Solid Edge part; units mm, degrees
sketch "Sketch1" plane through (0, 0, 0) normal (0, 0, 1) x (1, 0, 0)
  line L0 (-45.39, -6.825) -> (45.39, -6.825)
  line L1 (45.39, -6.825) -> (45.39, 6.825)
  line L2 (45.39, 6.825) -> (-45.39, 6.825)
  line L3 (-45.39, 6.825) -> (-45.39, -6.825)
  dimension "D1" = 45.39
  dimension "D2" = 45.39
extrude "Protrusion1" add sketch "Sketch1" along normal blind 1
sketch "Sketch2" plane through (0, 0, 1) normal (0, 0, 1) x (1, 0, 0)
  line L0 (-35.761, 0.4214) -> (-34.261, 0.4214)
  line L1 (-34.261, 0.4214) -> (-34.261, 6.4214)
  line L2 (-34.261, 6.4214) -> (-35.761, 6.4214)
  line L3 (-35.761, 6.4214) -> (-35.761, 0.4214)
  line L4 (-28.761, 0.4214) -> (-27.261, 0.4214)
  line L5 (-27.261, 0.4214) -> (-27.261, 6.4214)
  line L6 (-27.261, 6.4214) -> (-28.761, 6.4214)
  line L7 (-28.761, 6.4214) -> (-28.761, 0.4214)
  line L8 (-21.761, 0.3715) -> (-20.261, 0.3715)
  line L9 (-20.261, 0.3715) -> (-20.261, 6.3715)
  line L10 (-20.261, 6.3715) -> (-21.761, 6.3715)
  line L11 (-21.761, 6.3715) -> (-21.761, 0.3715)
  line L12 (-14.761, 0.3715) -> (-13.261, 0.3715)
  line L13 (-13.261, 0.3715) -> (-13.261, 6.3715)
  line L14 (-13.261, 6.3715) -> (-14.761, 6.3715)
  line L15 (-14.761, 6.3715) -> (-14.761, 0.3715)
  line L16 (-7.7611, 0.3715) -> (-6.2611, 0.3715)
  line L17 (-6.2611, 0.3715) -> (-6.2611, 6.3715)
  line L18 (-6.2611, 6.3715) -> (-7.7611, 6.3715)
  line L19 (-7.7611, 6.3715) -> (-7.7611, 0.3715)
  line L20 (-0.761, 0.3715) -> (0.739, 0.3715)
  line L21 (0.739, 0.3715) -> (0.739, 6.3715)
  line L22 (0.739, 6.3715) -> (-0.761, 6.3715)
  line L23 (-0.761, 6.3715) -> (-0.761, 0.3715)
  line L24 (-42.761, 0.4164) -> (-41.261, 0.4164)
  line L25 (-41.261, 0.4164) -> (-41.261, 6.4164)
  line L26 (-41.261, 6.4164) -> (-42.761, 6.4164)
  line L27 (-42.761, 6.4164) -> (-42.761, 0.4164)
  dimension "D1" = 41.261
  dimension "D2" = 41.261
  dimension "D3" = 34.261
  dimension "D4" = 34.261
  dimension "D5" = 27.261
  dimension "D6" = 27.261
  dimension "D7" = 20.261
  dimension "D8" = 20.261
  dimension "D9" = 13.261
  dimension "D10" = 13.261
  dimension "D11" = 6.2611
  dimension "D12" = 6.2611
  dimension "D13" = 0.739
  dimension "D14" = 0.739
extrude "Cutout1" cut sketch "Sketch2" against normal blind 0.5
mirror "Mirror1" about plane through (0, 0, 0) normal (1, 0, 0) of "Cutout1"
Source: CAD feature listing. Evaluate the final solid. Frame: model axes, mm. A direction names the side the tool comes from. Round coordinates to 2 decimals unless told otherwise and drop trailing zeros. Order: outer loops, then holes, each group sorted by start corner. A loop starts at its lowest first (then second) coordinate and runs counter-clockwise, first axis right, second up. Notation, with made-up numbers: (69, -36.5) -> (105, -36.5) arc R33 ccw to (105, 2.5) -> close; hole circle Ø5 at (84.5, -27). An arc over 180 degrees is marked (long way). One line per item, written item: value. Start each with the question number.
Q1. Section query A-A (x = -35). Return the cut outline in (y, z) (3 decimals).
Q2. Access query for faces 3 (the flat face through (-1, 0, 0)), 4 (the flat face through (-21, 3, 0.5)). Directions: +Z, -Z, +X, -X, +Y, -Y. A direction counts if a zero-diameter tool reaches every point of the face in a straight line with its end or side. Return the directions, or none.
Q3. Pin query (flat end, axial travel): pin 1 (1.2 mm diameter, centred on x = -14, y = 4.5, fed in from +Z). Return the tip coordinate at first contact, or that it passes through.
Q4. Material intervals for probe 1 along Y at (x, z) = (-7.5, 0.65) (1 decimal), sorted ascending.
Q5. Draft query along X for faces 1 (the flat face through (-1, 0, 1)), 2 (the flat face through (28, 3, 0.5)). Return one class per face: pulls with the +X half, pulls with the -X half, needs draft (parallel to the pull), parting line crosses it, or undercut.
Q6. Section query B-B (z = 0.75). Give the number of separate pieces and of enclosed holes in the cut face, plus the area to 3 significant figures.
Findings below:
1. outline: (-6.825, 0) -> (6.825, 0) -> (6.825, 1) -> (6.421, 1) -> (6.421, 0.5) -> (0.421, 0.5) -> (0.421, 1) -> (-6.825, 1) -> close
2. face 3: -Z, +X, -X, +Y, -Y
2. face 4: +Z
3. pin 1: z = 0.5
4. probe 1: -6.8 to 0.4, 6.4 to 6.8
5. face 1: needs draft
5. face 2: undercut
6. separate pieces: 1
6. enclosed holes: 13
6. area: 1,120 mm²
